Geometry: see drawing. Coordinates: mm, zero at the bounding-box minimum. Coordinates: 2 decimals unless noted, no trailing zeros. Order: outer loops, then holes, each group sorted by start corner. A loop starts at its lowest first (then second) coordinate and runs counter-clockwise, first axis right, second up.
Item 1: Section A-A on x = 56.5. Return the cut outline in (y, z).
Item 2: Ray query, line 1 (Z direction, x = 56.5, y = 0.4); line 2 (X direction, y = 0.7, z = 93.5); line 3 (X direction, y = 0.9, z = 91). Return the intervals inside material, ascending.
Item 3: Section D-D on x = 85. Return the cut outline in (y, z).
Item 4: Section C-C on y = 0.7. Return the cut outline in (x, z).
Item 5: Section B-B on z = 56.5. Return the cut outline in (x, y).
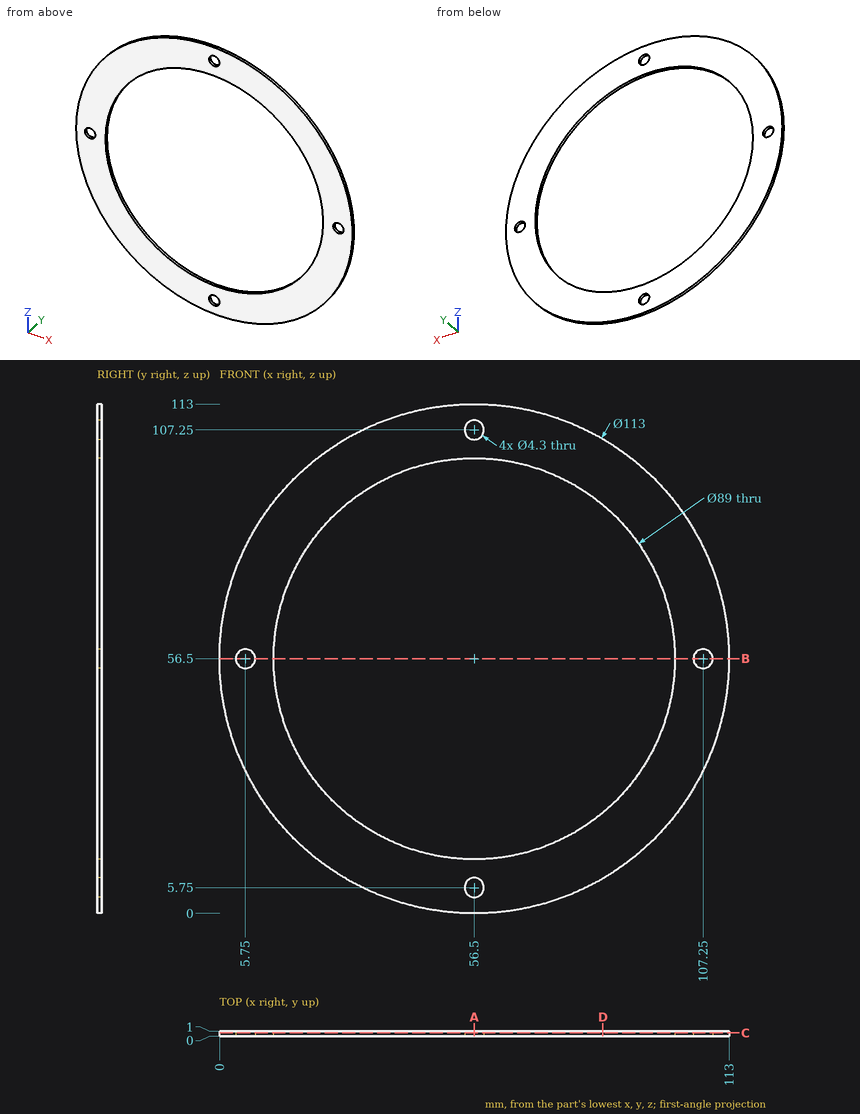
Answer list:
1. outline: (0, 0) - (1, 0) - (1, 3.6) - (0, 3.6) - close; (0, 7.9) - (1, 7.9) - (1, 12) - (0, 12) - close; (0, 101) - (1, 101) - (1, 105.1) - (0, 105.1) - close; (0, 109.4) - (1, 109.4) - (1, 113) - (0, 113) - close
2. line 1: z = 0 to 3.6, 7.9 to 12, 101 to 105.1, 109.4 to 113
2. line 2: x = 13.8 to 31.78, 81.22 to 99.2
2. line 3: x = 11.76 to 28.39, 84.61 to 101.24
3. outline: (0, 7.71) - (1, 7.71) - (1, 22.32) - (0, 22.32) - close; (0, 90.68) - (1, 90.68) - (1, 105.29) - (0, 105.29) - close
4. outline: circle Ø113 at (56.5, 56.5); hole circle Ø4.3 at (5.75, 56.5); hole circle Ø89 at (56.5, 56.5); hole circle Ø4.3 at (56.5, 5.75); hole circle Ø4.3 at (56.5, 107.25); hole circle Ø4.3 at (107.25, 56.5)
5. outline: (0, 0) - (3.6, 0) - (3.6, 1) - (0, 1) - close; (7.9, 0) - (12, 0) - (12, 1) - (7.9, 1) - close; (101, 0) - (105.1, 0) - (105.1, 1) - (101, 1) - close; (109.4, 0) - (113, 0) - (113, 1) - (109.4, 1) - close
